from build123d import *

# Parameters (mm, degrees)
F1_DEPTH = 40
F3_DEPTH = 25
F5_DEPTH = 25


with BuildPart() as f1:
    # F0 (on Right) → F1 (new body)
    with BuildSketch(Plane.YZ):
        Polygon((2.5, 4.3301270189), (0, 0), (5, 0), align=None)
    extrude(amount=F1_DEPTH)

    # F2 (on Top) → F3 (cut)
    with BuildSketch(Plane.XY):
        Polygon((0, 9.8450229721), (0, 0), (17.0520799894, 9.8450229721), align=None)
    extrude(amount=F3_DEPTH, mode=Mode.SUBTRACT)

    # F4 (on face) → F5 (cut)
    with BuildSketch(Plane(origin=(0, 0, 0), x_dir=(1, 0, 0), z_dir=(0, -0.8660254038, 0.5))):
        Polygon((0, 9.1414814892), (0, 0), (15.8335103958, 9.1414814892), align=None)
    extrude(amount=-F5_DEPTH, mode=Mode.SUBTRACT)

    # F7: F1 across plane


with BuildPart() as f1_1:
    add(f1.part)
    add(f1.part.mirror(Plane.YZ.offset(25)))


solid = f1_1.part
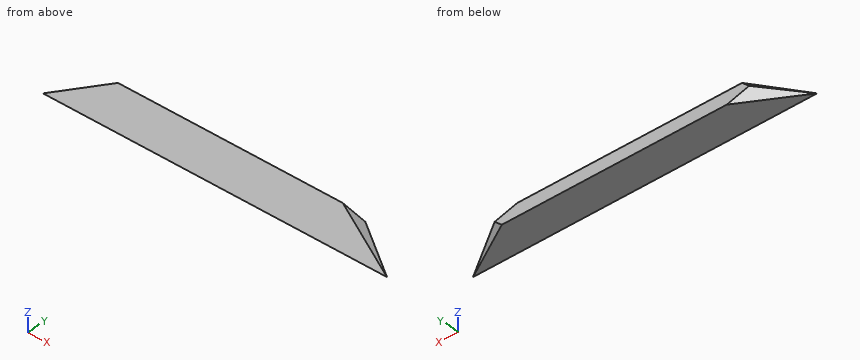
Part model, mm, in its own coordinate system. Coordinates: 2 decimals unless noted, no trailing zeros. Write each loop counter-clockwise with the first axis right and the second up, starting at its lowest first coordinate (ties: lowest second). Pieces come first, ordered by that corner, then holes. Notation, with made-up numbers: M 89.5,30.5 L 140.5,30.5 A23 ccw 140.5,45.5 Z; hole C 85.25,-35 d5. An arc over 180 degrees is marked long. Return JSON: item names as keys, results as strings.
1. Saw through at B-B, the plane z = 0.7. Write the cut outline in (x, y), then the cut area to 3 significant figures.
Determined:
{"outline": "M 1.4,0.4 L 48.6,0.4 L 47.9,1.21 L 42.04,4.6 L 7.96,4.6 L 2.1,1.21 Z", "area": "173 mm²"}
2. Saw through at A-A, the plane x = 28. Write the cut outline in (y, z).
Determined:
{"outline": "M 0,0 L 5,0 L 2.5,4.33 Z"}
3. Saw through at C-C, the plane y = 0.7. Write the cut outline in (x, z).
Determined:
{"outline": "M 1.21,0 L 48.79,0 L 48.79,0.4 L 47.58,1.21 L 2.42,1.21 L 1.21,0.4 Z"}
4. Saw through at D-D, the plane x = 43. Write the cut outline in (y, z), then the cut area to 3 significant figures.
Determined:
{"outline": "M 0,0 L 4.04,0 L 4.04,1.66 L 3.46,2.67 L 2.02,3.5 Z", "area": "9.23 mm²"}
5. Probe L1, parallel to Z at x = 17, y = 2.35; L2, parallel to Z at x = 34, y = 1.35; L3, parallel to Y at x = 5, z = 1.05. List the from-to ranges inside material, lowest first.
Determined:
{"L1": "0 to 4.07", "L2": "0 to 2.34", "L3": "0.61 to 2.89"}
